from build123d import *

# Parameters (mm, degrees)
SKETCH1_W                                         = 250
SKETCH1_H                                         = 150
BOSS_EXTRUDE1_DEPTH                               = 5
CUT_EXTRUDE1_DEPTH                                = 5
CSK_FOR_8_FLAT_HEAD_MACHINE_SCREW_100_D           = 4.4958
CSK_FOR_8_FLAT_HEAD_MACHINE_SCREW_100_CSINK_D     = 8.4328
CSK_FOR_8_FLAT_HEAD_MACHINE_SCREW_100_CSINK_ANGLE = 100
SKETCH4_W                                         = 10
SKETCH4_H                                         = 12.954582158
CUT_EXTRUDE2_DEPTH                                = 10


with BuildPart() as part:
    # Sketch1 → Boss-Extrude1 (new body)
    with BuildSketch(Plane(origin=(0, 0, 0), x_dir=(1, 0, 0), z_dir=(0, 1, 0))):
        with Locations((125, 75)):
            Rectangle(SKETCH1_W, SKETCH1_H)
    extrude(amount=BOSS_EXTRUDE1_DEPTH)

    # Sketch2 → Cut-Extrude1 (cut)
    with BuildSketch(Plane(origin=(0, 5, 0), x_dir=(1, 0, 0), z_dir=(0, 1, 0))):
        Polygon((5, 5), (245, 5), (245, 68.522708921), (235, 68.522708921), (235, 81.477291079), (245, 81.477291079), (245, 145), (5, 145), align=None)
    extrude(amount=-CUT_EXTRUDE1_DEPTH, mode=Mode.SUBTRACT)

    # CSK for #8 Flat Head Machine Screw (100)1 (through all)
    with Locations(Plane(origin=(240.110859841, 5, -75.135992341), x_dir=(0, 0, 1), z_dir=(0, 1, 0))):
        with Locations((0, 0)):
            CounterSinkHole(CSK_FOR_8_FLAT_HEAD_MACHINE_SCREW_100_D / 2, CSK_FOR_8_FLAT_HEAD_MACHINE_SCREW_100_CSINK_D / 2, counter_sink_angle=CSK_FOR_8_FLAT_HEAD_MACHINE_SCREW_100_CSINK_ANGLE)

    # Sketch4 → Cut-Extrude2 (cut)
    with BuildSketch(Plane(origin=(0, 5, 0), x_dir=(1, 0, 0), z_dir=(0, 1, 0))):
        with Locations((240, 75)):
            Rectangle(SKETCH4_W, SKETCH4_H)
    extrude(amount=-CUT_EXTRUDE2_DEPTH, mode=Mode.SUBTRACT)


solid = part.part
Design review of the part built by this model. Coordinates are the model's own, in mm. A direction names the side the tool comes from. Give positions to 0.01 mm unless a question says otherwise; leave off trailing zeros. Loops run counter-clockwise (first coordinate to the right, second up) from the corner with the lowest first, then second, coordinate; pieces in that order, holes last. Notation, with made-up numbers: M -27,-18 L 3,-18 A22 ccw 3,-2 Z; hole C -19,48 d6. An arc over 180 degrees is marked long. Write item = value, one per line.
Q1. For faces 4 (the flat face through (123, 2, 0)), 5 (the flat face through (5, 3, -76)), list the 3-axis set-ups (+Z, -Z, +X, -X, +Y, -Y) from which the entire face can be reached by the end or side of a thin tool; tool diameter is ignored.
Output values:
face_4 = +Z, +X, -X, +Y, -Y
face_5 = +Y, -Y
Q2. To check wall thickness, follow line 1 (Z direction, x = 168, y = 0.5); line 2 (X direction, y = 3.9, z = -107.5). State the ranges of each line that lie inside material, in increasing order. Write a range as [from, to].
Output values:
line_1 = [-150, -145], [-5, 0]
line_2 = [0, 5], [245, 250]
Q3. We need section B-B (z = -101). Give the boundary of the cut face in (x, y).
Output values:
outline = M 0,0 L 5,0 L 5,5 L 0,5 Z; M 245,0 L 250,0 L 250,5 L 245,5 Z
Q4. We need section C-C (x = 78). Give the boundary of the cut face in (y, z).
Output values:
outline = M 0,-150 L 5,-150 L 5,-145 L 0,-145 Z; M 0,-5 L 5,-5 L 5,0 L 0,0 Z
Q5. Draft analysis for pull direction X (two halves, no side actions). For faces 1 (the flat face through (87, 5, -3)), 2 (the flat face through (250, 2, -74)), 3 (the flat face through (245, 3, -74)), state which applies: +X half, -X half, draft (parallel to the pull), parting line (faces both ways), or undercut.
Output values:
face_1 = draft
face_2 = +X half
face_3 = undercut
Q6. We need section A-A (y = 1.7). Give the boundary of the cut face in (x, z), plus the area to 3 significant figures.
Output values:
outline = M 0,-150 L 250,-150 L 250,0 L 0,0 Z; hole M 5,-145 L 245,-145 L 245,-5 L 5,-5 Z
area = 3,900 mm^2
